Model file for the job. Use its own axes, mm. A direction names the side the tool comes from. Give positions to 0.01 mm unless a question says otherwise; leave off trailing zeros. Order: outer loops, then holes, each group sorted by start corner. A loop starts at its lowest first (then second) coordinate and runs counter-clockwise, first axis right, second up. Notation, with made-up numbers: (74.25, 6.25) -> (81.25, 6.25) arc R24 ccw to (81.25, 32.25) -> close; hole circle Ø9 at (81.5, -18). An arc over 180 degrees is marked (long way). Use CSV: the item, a comma, the result in double quotes. Start each with the question number.
1. Pull direction X, two halves, no side cores. Call faces 3 (the cylindrical face through (9.55, -0.27, 15.01)), 4 (the conical face through (15, -25, 0)), 5 (the cylindrical face through (18.8, -16.42, -2.11)): released by +X, released by -X, zero draft, split by the parting line, or undercut.
2. Cut at D-D on z = 0. Give the number of separate pieces and of enclosed holes in the cut face, then the cut area to 3 significant figures.
3. Cut at B-B on y = 0. List the corners of the cut face in (x, z), then the cut area to 3 significant figures.
4. Cut at A-A on x = 7.5. List the corners of the cut face in (y, z).
5. Drop flat-ended pins along their axis: pin 1 (6 mm diameter, centred on y = 5.5, z = -6, fed in from +X); pin 2 (6.5 mm diameter, centred on y = 21.5, z = 0, fed in from -X); pin 3 (5.5 mm diameter, centred on y = 22.5, z = -1, fed in from +X); pin 4 (3 mm diameter, centred on x = 6.5, z = 13, fed in from -Y). Give the stop position or say it passes through.
6. Cut at C-C on x = 12.25. List the corners of the cut face in (y, z), then the cut area to 3 significant figures.
7. Wall check: line 1 (X direction, y = 0, z = -16.75); line 2 (Z direction, x = 11.5, y = 0.5); line 3 (Z direction, x = 16, y = 0). Give the ranges that are in metal, low to high. Write a range as from..to.
8. 3-axis set-ups, long thin cutter, end or side, ignore diameter. For faces 1 (the cylindrical face through (18.056, 6.691, -12.864)), 2 (the flat face through (11, 0, 20)): which of +Z, -Z, +X, -X, +Y, -Y reach the whole face in a straight line?
Autodesk Inventor part; units mm, degrees
ref_plane "to_bearings_XY" through (14, 0, 0) normal (1, 0, 0) x (0, 0, -1)
ref_plane "to_bearings_YZ" through (14, 0, 0) normal (0, 0, -1) x (0, 1, 0)
ref_plane "to_bearings_ZX" through (14, 0, 0) normal (0, 1, 0) x (1, 0, 0)
sketch "Sketch_1" plane through (0, 0, 0) normal (0, 0, 1) x (1, 0, 0)
  line L0 (22, 0) -> (0, 0)
  line L1 (0, 28) -> (0, 10.5)
  line L2 (0, 10.5) -> (14, 10.5)
  line L3 (14, 10.5) -> (14, 14.5)
  line L4 (14, 14.5) -> (22, 14.5)
  line L5 (22, 14.5) -> (22, 28)
  line L6 (22, 28) -> (0, 28)
revolve "Revolution1" add sketch "Sketch_1" angle 360 about axis through (22, 0, 0) along (1, 0, 0)
sketch "Sketch_2" plane through (0, 0, 0) normal (1, 0, 0) x (0, 1, 0)
  line L0 (-112, 80) -> (-112, -80)
  line L1 (-112, -80) -> (112, -80)
  line L2 (112, -80) -> (112, 80)
  line L3 (112, 80) -> (-112, 80)
  line L4 (-28, 20) -> (-28, -20)
  line L5 (-28, -20) -> (28, -20)
  line L6 (28, -20) -> (28, 20)
  line L7 (28, 20) -> (-28, 20)
extrude "Extrusion1" cut sketch "Sketch_2" along normal blind 24
sketch "Sketch_3" plane through (0, 0, 0) normal (0, 0, 1) x (1, 0, 0)
  line L0 (22, 21.5) -> (0, 21.5)
  line L1 (0, 21.5) -> (0, 25.5)
  line L2 (0, 25.5) -> (0.6765, 24.8235)
  line L3 (0.6765, 24.8235) -> (14.8235, 24.8235)
  line L4 (14.8235, 24.8235) -> (15.5, 25.5)
  line L5 (15.5, 25.5) -> (15.5, 27)
  line L6 (15.5, 27) -> (22, 27)
  line L7 (22, 27) -> (22, 21.5)
  line L8 (22, 21.5) -> (0, 21.5)
revolve "Revolution2" cut sketch "Sketch_3" angle 360 about axis through (22, 21.5, 0) along (1, 0, 0)
thread "Thread1"
pattern_linear "Rectangular Pattern1" count 2 spacing 43 along (0, -1, 0) of "Revolution2"
sketch "Sketch_4" plane through (7.5, 0, 0) normal (1, 0, 0) x (0, 0, -1)
  line L0 (-10.15, 0) -> (-20, 0)
  line L1 (-20, 0) -> (-20, 2.5)
  line L2 (-20, 2.5) -> (-19.567, 2.067)
  line L3 (-19.567, 2.067) -> (-10.583, 2.067)
  line L4 (-10.583, 2.067) -> (-10.15, 2.5)
  line L5 (-10.15, 2.5) -> (-10.15, 0)
  line L6 (-10.15, 0) -> (-20, 0)
revolve "Revolution3" cut sketch "Sketch_4" angle 360 about axis through (7.5, 0, 10.15) along (0, 0, -1)
thread "Thread2"
sketch "Sketch_6" plane through (7.5, 0, 0) normal (1, 0, 0) x (0, 0, -1)
  line L0 (20, 0) -> (10.15, 0)
  line L1 (10.15, 0) -> (10.15, 2.5)
  line L2 (10.15, 2.5) -> (10.583, 2.067)
  line L3 (10.583, 2.067) -> (19.567, 2.067)
  line L4 (19.567, 2.067) -> (20, 2.5)
  line L5 (20, 2.5) -> (20, 0)
  line L6 (20, 0) -> (10.15, 0)
revolve "Revolution4" cut sketch "Sketch_6" angle 360 about axis through (7.5, 0, -20) along (0, 0, -1)
thread "Thread3"
ref_plane "to_bearings_XY" through (14, 0, 0) normal (1, 0, 0) x (0, 0, -1)
ref_plane "to_bearings_YZ" through (14, 0, 0) normal (0, 0, -1) x (0, 1, 0)
ref_plane "to_bearings_ZX" through (14, 0, 0) normal (0, 1, 0) x (1, 0, 0)
ref_plane "to_screw1_XY" through (7.5, 0, 10.5) normal (0, 0, 1) x (1, 0, 0)
ref_plane "to_screw1_YZ" through (7.5, 0, 10.5) normal (1, 0, 0) x (0, 1, 0)
ref_plane "to_screw1_ZX" through (7.5, 0, 10.5) normal (0, 1, 0) x (0, 0, 1)
ref_plane "to_screw2_XY" through (7.5, 0, -10.5) normal (0, 0, -1) x (1, 0, 0)
ref_plane "to_screw2_YZ" through (7.5, 0, -10.5) normal (1, 0, 0) x (0, -1, 0)
ref_plane "to_screw2_ZX" through (7.5, 0, -10.5) normal (0, -1, 0) x (0, 0, -1)
properties part number "BGCSB9_h"
Verdict:
1,face 3,"undercut"
1,face 4,"released by +X"
1,face 5,"zero draft"
2,separate pieces,"4"
2,enclosed holes,"0"
2,area,"355 mm^2"
3,outline,"(0, -20) -> (5, -20) -> (5.43, -19.57) -> (5.43, -10.58) -> (5.35, -10.5) -> (0, -10.5) -> close; (0, 10.5) -> (5.35, 10.5) -> (5.43, 10.58) -> (5.43, 19.57) -> (5, 20) -> (0, 20) -> close; (9.57, -19.57) -> (10, -20) -> (22, -20) -> (22, -14.5) -> (14, -14.5) -> (14, -10.5) -> (9.65, -10.5) -> (9.57, -10.58) -> close; (9.57, 10.58) -> (9.65, 10.5) -> (14, 10.5) -> (14, 14.5) -> (22, 14.5) -> (22, 20) -> (10, 20) -> (9.57, 19.57) -> close"
3,area,"275 mm^2"
4,outline,"(-19.6, -20) -> (-2.5, -20) -> (-2.07, -19.57) -> (-2.07, -10.58) -> (-2.44, -10.21) arc R10.5 cw to (-2.44, 10.21) -> (-2.07, 10.58) -> (-2.07, 19.57) -> (-2.5, 20) -> (-19.6, 20) arc R28 ccw to start; (2.07, -19.57) -> (2.5, -20) -> (19.6, -20) arc R28 ccw to (19.6, 20) -> (2.5, 20) -> (2.07, 19.57) -> (2.07, 10.58) -> (2.44, 10.21) arc R10.5 cw to (2.44, -10.21) -> (2.07, -10.58) -> close; hole circle Ø6.65 at (-21.5, 0); hole circle Ø6.65 at (21.5, 0)"
5,pin 1,"x = 14"
5,pin 2,"through"
5,pin 3,"x = 15.5"
5,pin 4,"y = -25.53"
6,outline,"(-19.6, -20) -> (19.6, -20) arc R28 ccw to (19.6, 20) -> (-19.6, 20) arc R28 ccw to start; hole circle Ø6.65 at (-21.5, 0); hole circle Ø21 at (0, 0); hole circle Ø6.65 at (21.5, 0)"
6,area,"1,620 mm^2"
7,line 1,"0..5.43, 9.57..22"
7,line 2,"-20..-10.49, 10.49..20"
7,line 3,"-20..-14.5, 14.5..20"
8,face 1,"+X"
8,face 2,"+Z, +X, -X, +Y, -Y"
